from build123d import *

# Parameters (mm, degrees)
BOSS_EXTRU_1_DEPTH      = 8
ESQUISSE2_R             = 20
ESQUISSE2_R_2           = 15
ENL_V_MAT_EXTRU_1_DEPTH = 4
ESQUISSE3_W             = 9.17
ESQUISSE3_H             = 20
BOSS_EXTRU_2_DEPTH      = 8
ESQUISSE7_W             = 6
ESQUISSE7_H             = 20
ENL_V_MAT_EXTRU_5_DEPTH = 6
ESQUISSE8_R             = 1.5
ENL_V_MAT_EXTRU_6_DEPTH = 10


with BuildPart() as part:
    # Esquisse1 → Boss.-Extru.1 (new body)
    with BuildSketch(Plane.XY):
        with BuildLine():
            Line((42.613906887, 3.786407767), (42.613906887, 23.786407767))
            Line((42.613906887, 23.786407767), (-43.211335831, 23.786407767))
            ThreePointArc((-43.211335831, 23.786407767), (-29.069200208, 17.928543391), (-23.211335831, 3.786407767))
            Line((-23.211335831, 3.786407767), (42.613906887, 3.786407767))
        make_face()
        with BuildLine():
            ThreePointArc((-23.211335831, 3.786407767), (-29.069200208, 17.928543391), (-43.211335831, 23.786407767))
            Line((-43.211335831, 23.786407767), (-43.211335831, 18.786407767))
            ThreePointArc((-43.211335831, 18.786407767), (-32.604734113, 14.393009485), (-28.211335831, 3.786407767))
            Line((-28.211335831, 3.786407767), (-23.211335831, 3.786407767))
        make_face()
        with BuildLine():
            Line((-43.211335831, 18.786407767), (-43.211335831, 23.786407767))
            ThreePointArc((-43.211335831, 23.786407767), (-57.353471455, -10.355727857), (-23.211335831, 3.786407767))
            Line((-23.211335831, 3.786407767), (-28.211335831, 3.786407767))
            ThreePointArc((-28.211335831, 3.786407767), (-53.817937549, -6.820193951), (-43.211335831, 18.786407767))
        make_face()
    extrude(amount=BOSS_EXTRU_1_DEPTH)

    # Esquisse2 → Enlèv. mat.-Extru.1 (cut)
    with BuildSketch(Plane.XY.offset(8)):
        with Locations((-43.211335831, 3.786407767)):
            Circle(ESQUISSE2_R)
        with Locations((-43.211335831, 3.786407767)):
            Circle(ESQUISSE2_R_2, mode=Mode.SUBTRACT)
    extrude(amount=-ENL_V_MAT_EXTRU_1_DEPTH, mode=Mode.SUBTRACT)

    # Esquisse3 → Boss.-Extru.2 (add)
    with BuildSketch(Plane.XY.offset(8)):
        with Locations((47.198906887, 13.786407767)):
            Rectangle(ESQUISSE3_W, ESQUISSE3_H)
    extrude(amount=-BOSS_EXTRU_2_DEPTH)

    # Esquisse7 → Enlèv. mat.-Extru.5 (cut)
    with BuildSketch(Plane.XY.offset(8)):
        with Locations((48.783906887, 13.786407767)):
            Rectangle(ESQUISSE7_W, ESQUISSE7_H)
    extrude(amount=-ENL_V_MAT_EXTRU_5_DEPTH, mode=Mode.SUBTRACT)

    # Esquisse8 → Enlèv. mat.-Extru.6 (cut)
    with BuildSketch(Plane.XY.offset(8)):
        with Locations((-26.216093113, 21.786407767)):
            Circle(ESQUISSE8_R)
        with Locations((-11.216093113, 21.786407767)):
            Circle(ESQUISSE8_R)
    extrude(amount=-ENL_V_MAT_EXTRU_6_DEPTH, mode=Mode.SUBTRACT)


solid = part.part
Design review of the part built by this model. Coordinates are the model's own, in mm. A direction names the side the tool comes from. Give positions to 0.01 mm unless a question says otherwise; leave off trailing zeros. Loops run counter-clockwise (first coordinate to the right, second up) from the corner with the lowest first, then second, coordinate; pieces in that order, holes last. Notation, with made-up numbers: (58.5, -38.75) -> (86.5, -38.75) arc R26 cw to (86.5, -14.75) -> close; hole circle Ø11 at (21, 41.5). An arc over 180 degrees is marked (long way). One line per question, with ' | ' between items. Start each with the question number.
(1) We need section B-B (x = -55.5). State the section outline as (y, z) points.
(2) We need section C-C (x = -3). State the section outline as (y, z) points.
(3) Insertion check: P1, Ø6.5, axis at x = 49, y = 11.5, coming from the +Z side; P2, Ø1.5, axis at y = 18.5, z = 2, coming from the -X side; P3, Ø1, axis at y = 7.5, z = 1.5, coming from the -X side; P4, Ø1.8, axis at y = 9, z = 4, coming from the +X side. Each pin has a flat end and moves straight along its axis. Give the tip position at first contact, or say it passes through.
(4) For line 1 (X direction, y = 4, z = 3); line 2 (Y direction, x = 4.5, z = 4.75); line 3 (X direction, y = 4, z = 1.75), list the stretches that pass through material, from the lowest coordinate up.
(5) For faces 4 (the face through (45.784, 14, 5)), 5 (the face through (-28.91, 17.77, 6.03)), 6 (the face through (4, 23.786, 4)), list the 3-axis set-ups (+Z, -Z, +X, -X, +Y, -Y) from which the entire face can be reached by the end or side of a thin tool; tool diameter is ignored.
(6) We need section D-D (z = 7). State the section outline as (x, y) points, and give its area (3 significant figures).
(7) Draft analysis for pull direction Y (two halves, no side actions). For faces 1 (the face through (-9.83, 21.21, 4.06)), 2 (the face through (-7, 13, 0)), 3 (the face through (14, 3.786, 4)), state which applies: +Y half, -Y half, draft (parallel to the pull), parting line (faces both ways), or undercut.
(8) We need section A-A (y = 8). State the section outline as (x, z) points.
The answers:
1) outline: (-11.99, 0) -> (-4.82, 0) -> (-4.82, 4) -> (-11.99, 4) -> close; (12.39, 0) -> (19.57, 0) -> (19.57, 4) -> (12.39, 4) -> close
2) outline: (3.79, 0) -> (23.79, 0) -> (23.79, 8) -> (3.79, 8) -> close
3) P1: stops at z = 8 | P2: stops at x = -57.53 | P3: stops at x = -62.95 | P4: stops at x = 45.78
4) line 1: x = -63.21 to -58.21, -28.21 to 45.78 | line 2: y = 3.79 to 23.79 | line 3: x = -63.21 to -58.21, -28.21 to 51.78
5) face 4: +Z, +X, +Y, -Y | face 5: +Z, -X, -Y | face 6: +Z, -Z, +X, -X, +Y
6) outline: (-43.21, 23.79) arc R20 cw to (-23.21, 3.79) -> (45.78, 3.79) -> (45.78, 23.79) -> close; hole circle Ø3 at (-26.22, 21.79); hole circle Ø3 at (-11.22, 21.79) | area: 1,450 mm^2
7) face 1: undercut | face 2: draft | face 3: -Y half
8) outline: (-62.76, 0) -> (-57.61, 0) -> (-57.61, 4) -> (-62.76, 4) -> close; (-28.82, 0) -> (51.78, 0) -> (51.78, 2) -> (45.78, 2) -> (45.78, 8) -> (-23.66, 8) -> (-23.66, 4) -> (-28.82, 4) -> close
